For this review, use the dimensioned drawing (mm, ordinates from the lowest corner) and the shaded views. Coordinates: 2 decimals unless noted, no trailing zeros. Write each loop counter-clockwise with the first axis right and the second up, starting at its lowest first coordinate (ties: lowest second). Pieces come first, ordered by that corner, then holes. Notation, with made-up numbers: M 15,30.5 L 26,30.5 A14 ccw 26,56.5 Z; hole C 55.5,-20.75 d5. An arc over 180 degrees is marked long. Return JSON: item names as keys, results as strings.
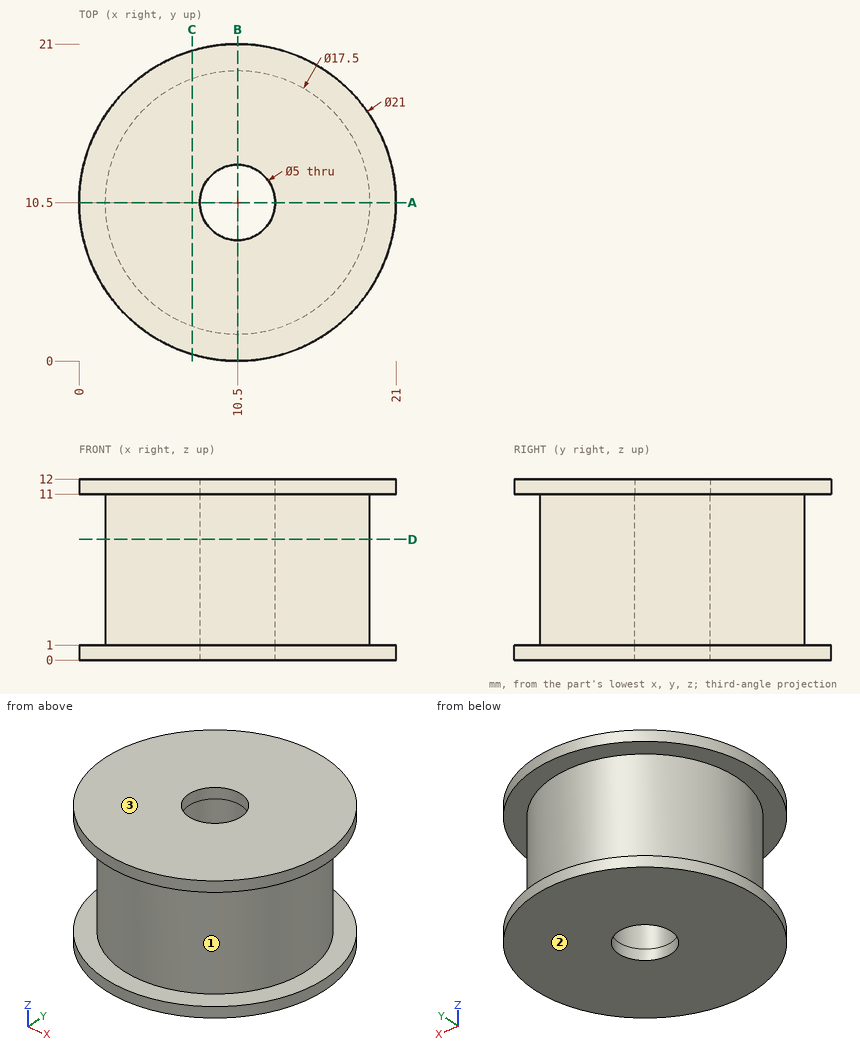
1. Draft analysis for pull direction Z (two halves, no side actions). For the marked faces 1, 2 and 3, state which applies: +Z half, -Z half, draft (parallel to the pull), parting line (faces both ways), or undercut.
Checks:
{"face 1": "undercut", "face 2": "-Z half", "face 3": "+Z half"}
2. We need section C-C (x = 7.5). State the section outline as (y, z) points.
Checks:
{"outline": "M 0.44,0 L 20.56,0 L 20.56,1 L 18.72,1 L 18.72,11 L 20.56,11 L 20.56,12 L 0.44,12 L 0.44,11 L 2.28,11 L 2.28,1 L 0.44,1 Z"}
3. We need section A-A (y = 10.5). State the section outline as (x, z) points, plus the area to 3 significant figures.
Checks:
{"outline": "M 0,0 L 8,0 L 8,12 L 0,12 L 0,11 L 1.75,11 L 1.75,1 L 0,1 Z; M 13,0 L 21,0 L 21,1 L 19.25,1 L 19.25,11 L 21,11 L 21,12 L 13,12 Z", "area": "157 mm2"}
4. Clearance check with flat-ended pins moving along their axes: pin 1 Ø2 at (x, z) = (2.5, 9) entering from +Y; pin 2 Ø2 at (x, z) = (15, 8) entering from +Y; pin 3 Ø3 at (x, z) = (7.5, 2) entering from -Y. State where each tip first meets the part, or that it passes through.
Checks:
{"pin 1": "y = 15.75", "pin 2": "y = 18.52", "pin 3": "y = 0.17"}
5. Wall thickness on L1, parallel to Y at x = 10.5, z = 0.75; L2, parallel to Z at x = 1.75, y = 7.5; L3, parallel to Y at x = 10.5, z = 7.5: over which ranges is each line inside the solid? List them lowest first. Write a range as from..to.
Checks:
{"L1": "0..8, 13..21", "L2": "0..1, 11..12", "L3": "1.75..8, 13..19.25"}
6. We need section D-D (z = 8). State the section outline as (x, y) points.
Checks:
{"outline": "C 10.5,10.5 d17.5; hole C 10.5,10.5 d5"}
